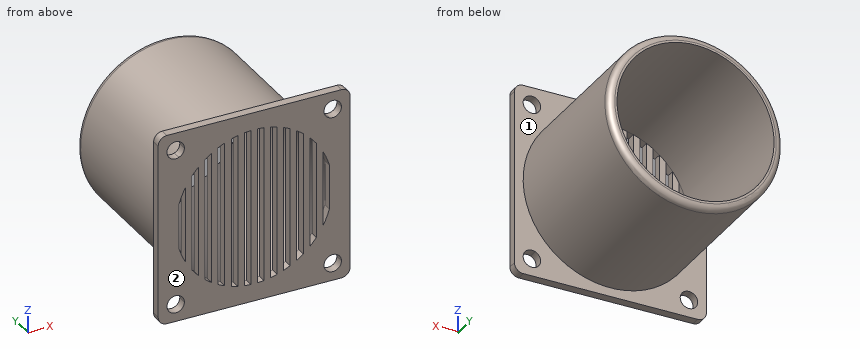
from build123d import *
from build123d.topology import SkipClean

# Parameters (mm, degrees)
ESBO_O1_W                = 44
ESBO_O1_H                = 44
RESSALTO_EXTRUS_O1_DEPTH = 2
ESBO_O3_R                = 20
ESBO_O3_R_2              = 18
RESSALTO_EXTRUS_O3_DEPTH = 37
FILETE3_R                = 1.5
FILETE4_R                = 2


with BuildPart() as part:
    # Esboço1 → Ressalto-extrusão1 (new body)
    with BuildSketch(Plane(origin=(0, 0, 0), x_dir=(1, 0, 0), z_dir=(0, 1, 0))):
        Rectangle(ESBO_O1_W, ESBO_O1_H)
        with BuildLine():
            ThreePointArc((-16, -18), (-19.658312395, -19.118033989), (-17.25, -16.145950378))
            ThreePointArc((-17.25, -16.145950378), (-16.341687605, -16.881966011), (-16, -18))
        make_face(mode=Mode.SUBTRACT)
        with BuildLine():
            ThreePointArc((-3.75, -17.605041891), (-4.50417298, -17.427347066), (-5.25, -17.217360425))
            Line((-5.25, -17.217360425), (-5.25, 17.217360425))
            ThreePointArc((-5.25, 17.217360425), (-4.50417298, 17.427347066), (-3.75, 17.605041891))
            Line((-3.75, 17.605041891), (-3.75, -17.605041891))
        make_face(mode=Mode.SUBTRACT)
        with BuildLine():
            ThreePointArc((20, -18), (16.881966011, -19.658312395), (17.25, -16.145950378))
            ThreePointArc((17.25, -16.145950378), (19.118033989, -16.341687605), (20, -18))
        make_face(mode=Mode.SUBTRACT)
        with BuildLine():
            ThreePointArc((-15.75, -8.714212529), (-16.596404379, -6.968454757), (-17.25, -5.14174095))
            Line((-17.25, -5.14174095), (-17.25, 5.14174095))
            ThreePointArc((-17.25, 5.14174095), (-16.596404379, 6.968454757), (-15.75, 8.714212529))
            Line((-15.75, 8.714212529), (-15.75, -8.714212529))
        make_face(mode=Mode.SUBTRACT)
        with BuildLine():
            ThreePointArc((-12.75, -12.70580576), (-13.527005163, -11.875189739), (-14.25, -10.997158724))
            Line((-14.25, -10.997158724), (-14.25, 10.997158724))
            ThreePointArc((-14.25, 10.997158724), (-13.527005163, 11.875189739), (-12.75, 12.70580576))
            Line((-12.75, 12.70580576), (-12.75, -12.70580576))
        make_face(mode=Mode.SUBTRACT)
        with BuildLine():
            ThreePointArc((-9.75, -15.130680751), (-10.513862046, -14.610226038), (-11.25, -14.051245496))
            Line((-11.25, -14.051245496), (-11.25, 14.051245496))
            ThreePointArc((-11.25, 14.051245496), (-10.513862046, 14.610226038), (-9.75, 15.130680751))
            Line((-9.75, 15.130680751), (-9.75, -15.130680751))
        make_face(mode=Mode.SUBTRACT)
        with BuildLine():
            ThreePointArc((-6.75, -16.686446596), (-7.507894085, -16.359447619), (-8.25, -15.998046756))
            Line((-8.25, -15.998046756), (-8.25, 15.998046756))
            ThreePointArc((-8.25, 15.998046756), (-7.507894085, 16.359447619), (-6.75, 16.686446596))
            Line((-6.75, 16.686446596), (-6.75, -16.686446596))
        make_face(mode=Mode.SUBTRACT)
        with BuildLine():
            Line((-0.75, 17.984368212), (-0.75, -17.984368212))
            ThreePointArc((-0.75, -17.984368212), (-1.501312927, -17.937281274), (-2.25, -17.85882135))
            Line((-2.25, -17.85882135), (-2.25, 17.85882135))
            ThreePointArc((-2.25, 17.85882135), (-1.501312927, 17.937281274), (-0.75, 17.984368212))
        make_face(mode=Mode.SUBTRACT)
        with BuildLine():
            ThreePointArc((-16, 18), (-16.341687605, 16.881966011), (-17.25, 16.145950378))
            ThreePointArc((-17.25, 16.145950378), (-19.658312395, 19.118033989), (-16, 18))
        make_face(mode=Mode.SUBTRACT)
        with BuildLine():
            ThreePointArc((2.25, -17.85882135), (1.501312927, -17.937281274), (0.75, -17.984368212))
            Line((0.75, -17.984368212), (0.75, 17.984368212))
            ThreePointArc((0.75, 17.984368212), (1.501312927, 17.937281274), (2.25, 17.85882135))
            Line((2.25, 17.85882135), (2.25, -17.85882135))
        make_face(mode=Mode.SUBTRACT)
        with BuildLine():
            ThreePointArc((5.25, -17.217360425), (4.50417298, -17.427347066), (3.75, -17.605041891))
            Line((3.75, -17.605041891), (3.75, 17.605041891))
            ThreePointArc((3.75, 17.605041891), (4.50417298, 17.427347066), (5.25, 17.217360425))
            Line((5.25, 17.217360425), (5.25, -17.217360425))
        make_face(mode=Mode.SUBTRACT)
        with BuildLine():
            ThreePointArc((8.25, -15.998046756), (7.507894085, -16.359447619), (6.75, -16.686446596))
            Line((6.75, -16.686446596), (6.75, 16.686446596))
            ThreePointArc((6.75, 16.686446596), (7.507894085, 16.359447619), (8.25, 15.998046756))
            Line((8.25, 15.998046756), (8.25, -15.998046756))
        make_face(mode=Mode.SUBTRACT)
        with BuildLine():
            ThreePointArc((11.25, -14.051245496), (10.513862046, -14.610226038), (9.75, -15.130680751))
            Line((9.75, -15.130680751), (9.75, 15.130680751))
            ThreePointArc((9.75, 15.130680751), (10.513862046, 14.610226038), (11.25, 14.051245496))
            Line((11.25, 14.051245496), (11.25, -14.051245496))
        make_face(mode=Mode.SUBTRACT)
        with BuildLine():
            ThreePointArc((14.25, -10.997158724), (13.527005163, -11.875189739), (12.75, -12.70580576))
            Line((12.75, -12.70580576), (12.75, 12.70580576))
            ThreePointArc((12.75, 12.70580576), (13.527005163, 11.875189739), (14.25, 10.997158724))
            Line((14.25, 10.997158724), (14.25, -10.997158724))
        make_face(mode=Mode.SUBTRACT)
        with BuildLine():
            ThreePointArc((17.25, -5.14174095), (16.596404379, -6.968454757), (15.75, -8.714212529))
            Line((15.75, -8.714212529), (15.75, 8.714212529))
            ThreePointArc((15.75, 8.714212529), (16.596404379, 6.968454757), (17.25, 5.14174095))
            Line((17.25, 5.14174095), (17.25, -5.14174095))
        make_face(mode=Mode.SUBTRACT)
        with BuildLine():
            ThreePointArc((20, 18), (19.118033989, 16.341687605), (17.25, 16.145950378))
            ThreePointArc((17.25, 16.145950378), (16.881966011, 19.658312395), (20, 18))
        make_face(mode=Mode.SUBTRACT)
    extrude(amount=RESSALTO_EXTRUS_O1_DEPTH)

    # Esboço3 → Ressalto-extrusão3 (add)
    with SkipClean():  # the faces are left unmerged after this step: merging them gives an invalid solid
        with BuildSketch(Plane(origin=(0, 2, 0), x_dir=(1, 0, 0), z_dir=(0, 1, 0))):
            with Locations(Location((0, 0, 0), (0, 0, 270))):
                Circle(ESBO_O3_R)
            with Locations(Location((0, 0, 0), (0, 0, 87.611984537))):
                Circle(ESBO_O3_R_2, mode=Mode.SUBTRACT)
        extrude(amount=RESSALTO_EXTRUS_O3_DEPTH)

    # Filete3
    filete3_edges = [part.edges().sort_by_distance(p)[0] for p in [
        (0, 39, -20),
    ]]
    fillet(filete3_edges, radius=FILETE3_R)

    # Filete4
    filete4_edges = [part.edges().sort_by_distance(p)[0] for p in [
        (-22, 1, 22),
        (-22, 1, -22),
        (22, 1, -22),
        (22, 1, 22),
    ]]
    fillet(filete4_edges, radius=FILETE4_R)


solid = part.part
Here's how the part is built. I have some questions about the finished solid (model axes, mm). Face numbers are marked on the shaded views. A direction names the side the tool comes from. Give positions to 0.01 mm unless a question says otherwise; leave off trailing zeros. Write each loop counter-clockwise with the first axis right and the second up, starting at its lowest first coordinate (ties: lowest second). Pieces come first, ordered by that corner, then holes. Notation, with made-up numbers: (66.5, 39.25) -> (80.5, 39.25) arc R18 cw to (80.5, 45.25) -> close; hole circle Ø11 at (-17, -2). An arc over 180 degrees is marked (long way). Use one line per item in the form item = value. Start each with the question number.
1. Will these pins go through, and if not, where does the flat tip stop? pin 1 Ø0.6 at (x, z) = (-17.5, -2) entering from +Y; pin 2 Ø6 at (y, z) = (30.5, -10) entering from -X (3 decimals); pin 3 Ø10 at (y, z) = (18.5, 8.5) entering from +X.
2. If I drill on L1, parallel to Z at x = -18, y = 1; L2, parallel to X at y = 24, z = 0; L3, parallel to Z at x = 0.5, y = 26.5, over which ranges is the centre line in solid material (lowest first)?
3. Imagine slicing it at A-A on z = 0. State how many separate pieces and enclosed holes the cut face has, plus the area to 3 significant figures.
4. Imagine slicing it at B-B on y = 16.5. List the corners of the cut face in (x, z) for me.
5. On a 3-axis mill with a long thin cutter (end or side, diameter ignored), from which of +Z, -Z, +X, -X, +Y, -Y can I reach the whole of each face in a straight line? I mean the marked faces 1 and 2. Say none if no direction works.
Entries:
q1.pin_1 = 2
q1.pin_2 = -18.735
q1.pin_3 = 19.69
q2.L1 = -22 to -20, -16 to 16, 20 to 22
q2.L2 = -20 to -18, 18 to 20
q2.L3 = -19.99 to -17.99, 17.99 to 19.99
q3.separate_pieces = 13
q3.enclosed_holes = 0
q3.area = 199 mm²
q4.outline = circle Ø40 at (0, 0); hole circle Ø36 at (0, 0)
q5.face_1 = +Y
q5.face_2 = +Z, -Z, +X, -X, -Y
